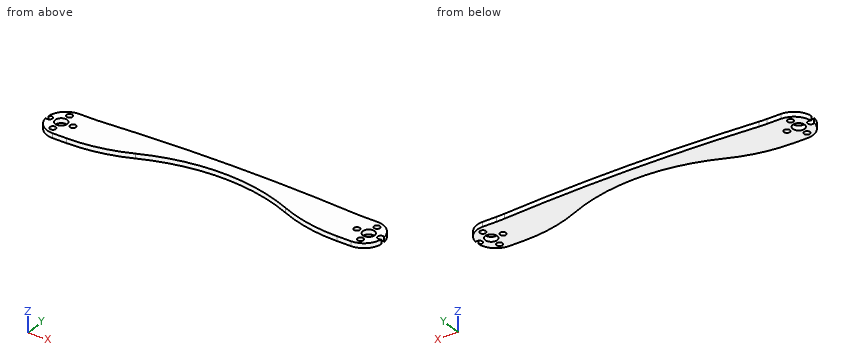
from build123d import *

# Parameters (mm, degrees)
BOSS_EXTRUDE1_DEPTH = 3.175
SKETCH3_R           = 1.984375
SKETCH3_R_2         = 4
CUT_EXTRUDE1_DEPTH  = 4.175


with BuildPart() as part:
    # Sketch2 → Boss-Extrude1 (new body)
    with BuildSketch(Plane.XY):
        with BuildLine():
            Line((0, 12.7), (9.464409507, 12.7))
            ThreePointArc((9.464409507, 12.7), (12.110944898, 12.745972855), (14.754286883, 12.883835947))
            ThreePointArc((14.754286883, 12.883835947), (100.825000026, 15.875), (186.895713169, 12.883835947))
            ThreePointArc((186.895713169, 12.883835947), (189.539055154, 12.745972855), (192.185590545, 12.7))
            Line((192.185590545, 12.7), (201.650000052, 12.7))
            ThreePointArc((201.650000052, 12.7), (214.350000052, 0), (201.650000052, -12.7))
            Line((201.650000052, -12.7), (192.185590545, -12.7))
            ThreePointArc((192.185590545, -12.7), (171.44657739, -10.560813054), (151.580883648, -4.233333333))
            ThreePointArc((151.580883648, -4.233333333), (100.825000026, 6.35), (50.069116404, -4.233333333))
            ThreePointArc((50.069116404, -4.233333333), (30.203422662, -10.560813054), (9.464409507, -12.7))
            Line((9.464409507, -12.7), (0, -12.7))
            ThreePointArc((0, -12.7), (-12.7, 0), (0, 12.7))
        make_face()
    extrude(amount=BOSS_EXTRUDE1_DEPTH)

    # Sketch3 → Cut-Extrude1 (cut, through all)
    with BuildSketch(Plane.XY.offset(3.175)):
        with Locations((-3.175, 8)):
            Circle(SKETCH3_R)
        with Locations((-3.175, 0)):
            Circle(SKETCH3_R_2)
        with Locations((204.825000052, 0)):
            Circle(SKETCH3_R_2)
        with Locations((204.825000052, 8)):
            Circle(SKETCH3_R)
        with Locations((212.825000052, 0)):
            Circle(SKETCH3_R)
        with Locations((204.825000052, -8)):
            Circle(SKETCH3_R)
        with Locations((196.825000052, 0)):
            Circle(SKETCH3_R)
        with Locations((4.825, 0)):
            Circle(SKETCH3_R)
        with Locations((-3.175, -8)):
            Circle(SKETCH3_R)
        with Locations((-11.175, 0)):
            Circle(SKETCH3_R)
    extrude(amount=-CUT_EXTRUDE1_DEPTH, mode=Mode.SUBTRACT)


solid = part.part
Verification items for the finished model (mm, model axes). Coordinates: 2 decimals unless noted, no trailing zeros. Order: outer loops, then holes, each group sorted by start corner. A loop starts at its lowest first (then second) coordinate and runs counter-clockwise, first axis right, second up. Notation, with made-up numbers: M 41,29 L 83,29 A25 cw 83,55 Z; hole C -9,4.25 d8. An arc over 180 degrees is marked long. Return JSON: item names as keys, results as strings.
1) Cross-section at A-A, the plane z = 1.4. Count the separate pieces of the cut face and the enclosed holes in it, and give its area (3 significant figures).
Answer list:
{"separate pieces": "1", "enclosed holes": "8", "area": "4,000 mm2"}
2) Gauge pin test, flat ends, axial feed: pin 1 (1.6 mm diameter, centred on x = 4.5, z = 2, fed in from +Y); pin 2 (3.5 mm diameter, centred on x = -3.175, y = -8, fed in from +Z). Record the tip position at first contact, or that the pin passes through.
Answer list:
{"pin 1": "y = 12.7", "pin 2": "through"}
3) Cross-section at C-C, the plane x = 106. Record the boundary of the cut face in (y, z) (3 decimals).
Answer list:
{"outline": "M 6.245,0 L 15.864,0 L 15.864,3.175 L 6.245,3.175 Z"}
4) Cross-section at D-D, the plane x = 71. Record the boundary of the cut face in (y, z) (3 decimals).
Answer list:
{"outline": "M 2.798,0 L 15.516,0 L 15.516,3.175 L 2.798,3.175 Z"}
5) Thickness scan on L1, parallel to X at y = 6.5, z = 3.05; L2, parallel to X at y = -4.25, z = 1; L3, parallel to Y at x = 7.5, z = 1.05. Record the ranges inside material, lowest first. Write a range as [from, to].
Answer list:
{"L1": "[-10.91, -4.47], [-1.88, 203.53], [206.12, 212.56]", "L2": "[-11.97, 50.03], [151.62, 213.62]", "L3": "[-12.7, 12.7]"}
6) Cross-section at B-B, the plane y = -8. Record the boundary of the cut face in (x, z) (3 decimals), and give its area (3 significant figures).
Answer list:
{"outline": "M -9.864,0 L -5.159,0 L -5.159,3.175 L -9.864,3.175 Z; M -1.191,0 L 40.009,0 L 40.009,3.175 L -1.191,3.175 Z; M 161.641,0 L 202.841,0 L 202.841,3.175 L 161.641,3.175 Z; M 206.809,0 L 211.514,0 L 211.514,3.175 L 206.809,3.175 Z", "area": "291 mm2"}
